Read the model definition and answer for the solid it produces. Units are mm, in the model's axes. Coordinates: 2 decimals unless noted, no trailing zeros. Loops run counter-clockwise (first coordinate to the right, second up) from the corner with the lowest first, then second, coordinate; pieces in that order, holes last. Notation, with made-up numbers: (12, 36.5) -> (48, 36.5) arc R13 ccw to (48, 47.5) -> close; hole circle Ø10 at (-19, 33). An arc over 180 degrees is marked (long way). Answer in a Markdown table with one row per item.
```python
from build123d import *

# Parameters (mm, degrees)
SKETCH1_R                       = 3.175
BOSS_EXTRUDE1_DEPTH             = 215
M4X0_7_TAPPED_HOLE1_D           = 3.3
M4X0_7_TAPPED_HOLE1_DEPTH       = 13.5
M4X0_7_TAPPED_HOLE1_CSINK_D     = 4
M4X0_7_TAPPED_HOLE1_CSINK_ANGLE = 90
M4X0_7_TAPPED_HOLE1_TIP         = 0.991420021
M4X0_7_TAPPED_HOLE2_D           = 3.3
M4X0_7_TAPPED_HOLE2_DEPTH       = 13.5
M4X0_7_TAPPED_HOLE2_CSINK_D     = 4
M4X0_7_TAPPED_HOLE2_CSINK_ANGLE = 90
M4X0_7_TAPPED_HOLE2_TIP         = 0.991420021
SKETCH7_W                       = 0.675
SKETCH7_H                       = 3
CHAMFER1_SIZE                   = 0.2


with BuildPart() as part:
    # Sketch1 → Boss-Extrude1 (new, symmetric)
    with BuildSketch(Plane.XY):
        Circle(SKETCH1_R)
    extrude(amount=BOSS_EXTRUDE1_DEPTH, both=True)

    # M4x0.7 Tapped Hole1
    with Locations(Plane(origin=(0, 0, -215), x_dir=(-1, 0, 0), z_dir=(0, 0, -1))):
        with Locations((0, 0)):
            CounterSinkHole(M4X0_7_TAPPED_HOLE1_D / 2, M4X0_7_TAPPED_HOLE1_CSINK_D / 2, depth=M4X0_7_TAPPED_HOLE1_DEPTH, counter_sink_angle=M4X0_7_TAPPED_HOLE1_CSINK_ANGLE)
            with Locations((0, 0, -(M4X0_7_TAPPED_HOLE1_DEPTH + M4X0_7_TAPPED_HOLE1_TIP / 2))):  # 118° drill point
                Cone(0, M4X0_7_TAPPED_HOLE1_D / 2, M4X0_7_TAPPED_HOLE1_TIP, mode=Mode.SUBTRACT)

    # M4x0.7 Tapped Hole2
    with Locations(Plane.XY.offset(215)):
        with Locations((0, 0)):
            CounterSinkHole(M4X0_7_TAPPED_HOLE2_D / 2, M4X0_7_TAPPED_HOLE2_CSINK_D / 2, depth=M4X0_7_TAPPED_HOLE2_DEPTH, counter_sink_angle=M4X0_7_TAPPED_HOLE2_CSINK_ANGLE)
            with Locations((0, 0, -(M4X0_7_TAPPED_HOLE2_DEPTH + M4X0_7_TAPPED_HOLE2_TIP / 2))):  # 118° drill point
                Cone(0, M4X0_7_TAPPED_HOLE2_D / 2, M4X0_7_TAPPED_HOLE2_TIP, mode=Mode.SUBTRACT)

    # Sketch7 → Cut-Revolve1 (revolve, cut)
    with BuildSketch(Plane(origin=(0, 0, 0), x_dir=(1, 0, 0), z_dir=(0, 1, 0)), mode=Mode.PRIVATE) as cut_revolve1_sk:
        with Locations((2.8375, 213.5)):
            Rectangle(SKETCH7_W, SKETCH7_H)
    revolve(cut_revolve1_sk.sketch.rotate(Axis((0, 0, -232.2463), (0, 0, 1)), 180), axis=Axis((0, 0, -232.2463), (0, 0, 1)), mode=Mode.SUBTRACT)

    # Chamfer1
    chamfer1_edges = [part.edges().sort_by_distance(p)[0] for p in [
        (2.5, 0, -215),
        (-3.175, 0, -212),
        (-3.175, 0, 215),
    ]]
    chamfer(chamfer1_edges, length=CHAMFER1_SIZE)


solid = part.part
```
1. Find the intervals of material crossed by probe 1 along Y at (x, z) = (0, 207.25) (3 decimals); probe 2 along X at (y, z) = (-0.25, -59); probe 3 along Z at (x, y) = (-2, -1.25), in increasing order.
A:
| item | result |
|---|---|
| probe 1 | y = -3.175 to -1.65, 1.65 to 3.175 |
| probe 2 | x = -3.17 to 3.17 |
| probe 3 | z = -214.94 to 215 |
2. Given pin 1 Ø1.5 at (x, z) = (1, 69.5) entering from -Y; pin 2 Ø1 at (x, z) = (2.5, 137) entering from -Y; pin 3 Ø2.5 at (x, y) = (0, 0) entering from +Z, each flat-ended and moving along its own axis, determine where each tip first touches the part or whether it passes through.
A:
| item | result |
|---|---|
| pin 1 | stops at y = -3.17 |
| pin 2 | stops at y = -2.47 |
| pin 3 | stops at z = 201.26 |
3. A cutting plane is placed at A-A on z = 147.5. Give the vertices of the cut face in (x, y) (3 decimals).
A:
| item | result |
|---|---|
| outline | circle Ø6.35 at (0, 0) |
